Autodesk Fusion 360 part; units mm, degrees
sketch "Sketch1" plane through (0, 0, 0) normal (0, 1, 0) x (1, 0, 0)
  circle A0 centre (0, 0) radius 23
  line L0 (-10, -15) -> (10, -15)
  line L1 (10, -15) -> (10, 15)
  line L2 (10, 15) -> (-10, 15)
  line L3 (-10, 15) -> (-10, -15)
  line L4 (1.75, 0) -> (22.5, 0) construction
  line L5 (0, -1.75) -> (0, -22.5) construction
  line L6 (-8, -14.25) -> (-12, -14.25)
  arc A1 (-12, -14.25) -> (-12, -15.75) centre (-12, -15) ccw
  line L7 (-12, -15.75) -> (-8, -15.75)
  arc A2 (-8, -15.75) -> (-8, -14.25) centre (-8, -15) ccw
  line L8 (-8, -15) -> (-12, -15) construction
  point P0 (-10, -15)
  point P1 (10, -15)
  point P2 (10, 15)
  point P3 (-10, 15)
  point P4 (-10, -15)
  point P5 (0, -17)
  dimension "d1" = 46
  dimension "d8" = 20
  dimension "d9" = 30
  dimension "d10" = 4
  dimension "d11" = 1.5
  dimension "d21" = 17
extrude "Extrude1" add sketch "Sketch1" along normal blind 10 contours A0 | L0 L3 L6 A2 | L0 L3 L6 A1 L7 A2 | L0 L1 L2 L3 L6 A2
hole "Hole1" at (0, 10, 0) direction (0, -1, 0) diameter 25 depth 9.5 tip angle 180
hole "Hole2" at (-10, 0, 15) direction (0, 1, 0) diameter 3.332 depth 5 tip angle 180
extrude "Extrude2" cut sketch "Sketch1" along normal blind 4 contours L0 L3 L6 A2 | L0 L3 L6 A1 L7 A2
pattern_linear "R-Pattern1" count 2 spacing 20 along (1, 0, 0) count 2 spacing 30 along (0, 0, -1) of "Extrude2", "Hole2"
sketch "Sketch2" plane through (0, 10, 0) normal (0, 1, 0) x (-1, 0, 0)
  circle A0 centre (0, 0) radius 12.5
  circle A1 centre (0, 0) radius 23
  point P0 (0, 17)
hole "Hole3" at (0, 10, 17) direction (0, -1, 0) diameter 3.332 depth 5 tip angle 180
pattern_circular "C-Pattern1" count 6 over 360 about axis through (0, 1.75, 0) along (0, 1, 0) of "Hole3"
Input: part model. Units: mm. Frame: model coordinates. A direction names the side the tool comes from. Give positions to 0.01 mm unless a question says otherwise; leave off trailing zeros. Order: outer loops, then holes, each group sorted by start corner. A loop starts at its lowest first (then second) coordinate and runs counter-clockwise, first axis right, second up. Notation, with made-up numbers: M 80.25,-11.75 L 94.25,-11.75 A19 cw 94.25,-0.75 Z; hole C 41,-0.75 d6. An arc over 180 degrees is marked long. Answer as a JSON object with one key per item and string values.
1. Cut plane D-D, the plane x = -10. Output: boundary loops of the cut face in (y, z).
Result sheet:
{"outline": "M 0,-20.71 L 10,-20.71 L 10,-7.5 L 0.5,-7.5 L 0.5,7.5 L 10,7.5 L 10,20.71 L 0,20.71 L 0,16.67 L 5,16.67 L 5,13.33 L 0,13.33 L 0,-13.33 L 5,-13.33 L 5,-16.67 L 0,-16.67 Z"}
2. Reachability of faces 1 (the cylindrical face through (16.374, 7.465, 8.717)), 2 (the cylindrical face through (9.5, 2.54, -16.59)) from +Z, -Z, +X, -X, +Y, -Y: full face, straight path, thin tool, end or side. Return the list, or none.
Result sheet:
{"face 1": "+Y", "face 2": "-Y"}
3. First-contact query: P1, Ø2, axis at x = 10, z = 15, coming from the -Y side; P2, Ø5, axis at y = 5, z = 12.5, coming from the -X side; P3, Ø2, axis at y = 1.5, z = -11.5, coming from the +X side. Flat tips, straight axial feed; report the tip coordinate or a pass-through.
Result sheet:
{"P1": "y = 5", "P2": "x = -20.71", "P3": "x = 20.46"}
4. Cut plane B-B, the plane z = 0. Output: boundary loops of the cut face in (x, y), and give its area (4 significant figures).
Result sheet:
{"outline": "M -23,0 L 23,0 L 23,10 L 12.5,10 L 12.5,0.5 L -12.5,0.5 L -12.5,10 L -23,10 Z", "area": "222.5 mm²"}
5. Pull-direction query (Z, two-part tool) for faces 3 (the cylindrical face through (-7.25, 1.97, 14.98)), 4 (the flat face through (0, 5, 17)), 5 (the flat face through (0, 0, 0)); classes: +Z half, -Z half, draft (parallel to the pull), parting line (faces both ways), or undercut.
Result sheet:
{"face 3": "undercut", "face 4": "undercut", "face 5": "draft"}
6. Cut plane A-A, the plane y = 2. State how many separate pieces and enclosed holes the cut face has, and give its area (3 significant figures).
Result sheet:
{"separate pieces": "1", "enclosed holes": "5", "area": "1,120 mm²"}
7. Ray query, line 1 (X direction, y = 7.7, z = 8.5); line 2 (Z direction, x = 0, y = 3.5); line 3 (Z direction, x = -10, y = 2). Return the intervals inside material, ascending. Write a range as [from, to].
Result sheet:
{"line 1": "[-21.37, -16.39], [-13.06, -9.17], [9.17, 13.06], [16.39, 21.37]", "line 2": "[-23, -12.5], [12.5, 23]", "line 3": "[-20.71, -16.67], [-13.33, -7.5], [7.5, 13.33], [16.67, 20.71]"}
8. Cut plane C-C, the plane y = 6.5. Output: boundary loops of the cut face in (x, z).
Result sheet:
{"outline": "C 0,0 d46; hole C -14.72,-8.5 d3.33; hole C -14.72,8.5 d3.33; hole C 0,0 d25; hole C 0,-17 d3.33; hole C 0,17 d3.33; hole C 14.72,-8.5 d3.33; hole C 14.72,8.5 d3.33"}
